CAD build for the part. Positions are in the model's coordinates, mm. Coordinates: 2 decimals unless noted, no trailing zeros. Answer in a Markdown table with one row per item. Add a question column.
Q1. Drill centre lines: line 1 along X through (y, z) = (1.45, 19); line 2 along Z through (x, y) = (18.5, 1.5); line 3 along Z through (x, y) = (45, 1.8). Where is each one in solid material? Low to high. Write a range as from..to.
Q2. Band-saw the part on A-A (y = 1.05). State how many separate pieces and enclosed holes the cut face has, and give its area (3 significant figures).
Q3. Pin check, flat tip, straight feed: pin 1 (0.6 mm diameter, centred on x = 13.1, z = -20, fed in from -Y). Stop position of the tip, or through.
```python
from build123d import *

# Parameters (mm, degrees)
SKETCH1_W             = 100
SKETCH1_H             = 50
BOSS_EXTRUDE1_DEPTH   = 2
FILLET1_R             = 6
F_3_0MM_DOWEL_HOLE1_D = 3
F_1_0MM_DOWEL_HOLE1_D = 1.02
LPATTERN1_COUNT       = 2
LPATTERN1_PITCH       = 2.54
LPATTERN1_COUNT_DIR2  = 20
LPATTERN1_PITCH_DIR2  = 2.54


with BuildPart() as part:
    # Sketch1 → Boss-Extrude1 (new body)
    with BuildSketch(Plane(origin=(0, 0, 0), x_dir=(1, 0, 0), z_dir=(0, 1, 0))):
        Rectangle(SKETCH1_W, SKETCH1_H)
    extrude(amount=BOSS_EXTRUDE1_DEPTH)

    # Fillet1
    fillet1_edges = [part.edges().sort_by_distance(p)[0] for p in [
        (50, 1, 25),
        (-50, 1, 25),
        (-50, 1, -25),
        (50, 1, -25),
    ]]
    fillet(fillet1_edges, radius=FILLET1_R)

    # Ø3.0mm Dowel Hole1 (through all)
    with Locations(Plane(origin=(-44, 2, -19), x_dir=(0, 0, 1), z_dir=(0, 1, 0))):
        with Locations((0, 0), (0, 88), (38, 88), (38, 0)):
            Hole(F_3_0MM_DOWEL_HOLE1_D / 2)

    # Ø1.0mm Dowel Hole1 (through all)
    with Locations(Plane(origin=(-25, 2, -20), x_dir=(0, 0, 1), z_dir=(0, 1, 0))):
        with Locations((0, 0)):
            f_1_0mm_dowel_hole1 = Hole(F_1_0MM_DOWEL_HOLE1_D / 2)

    # LPattern1: 1.0mm Dowel Hole1 2 × 20
    with Locations(*[(j * LPATTERN1_PITCH_DIR2, 0, i * LPATTERN1_PITCH) for i in range(LPATTERN1_COUNT) for j in range(LPATTERN1_COUNT_DIR2) if (i, j) != (0, 0)]):
        add(f_1_0mm_dowel_hole1, mode=Mode.SUBTRACT)


solid = part.part
```
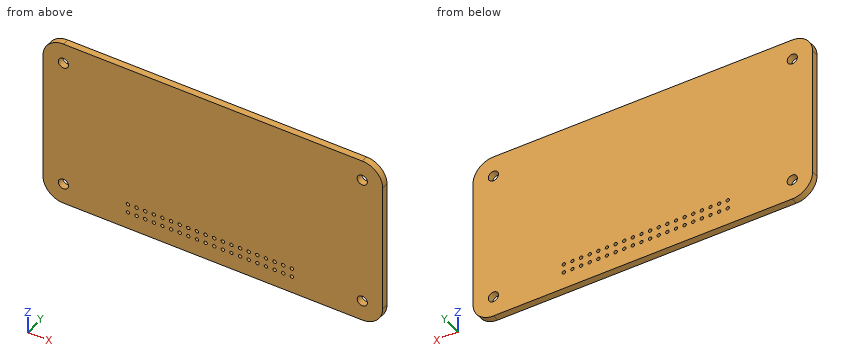
Checked values:
| question | item | result |
|---|---|---|
| 1 | line 1 | x = -50..-45.5, -42.5..42.5, 45.5..50 |
| 1 | line 2 | z = -25..-20.4, -19.6..-17.86, -17.06..25 |
| 1 | line 3 | z = -24.92..-20.12, -17.88..17.88, 20.12..24.92 |
| 2 | separate pieces | 1 |
| 2 | enclosed holes | 44 |
| 2 | area | 4,910 mm² |
| 3 | pin 1 | passes through |
